Here's the drawing with two shaded views (mm, measured from the low corner). I have some questions. A direction names the side the tool comes from. Round coordinates to 2 decimals unless told otherwise and drop trailing zeros. Loops run counter-clockwise (first coordinate to the right, second up) from the corner with the lowest first, then second, coordinate; pieces in that order, holes last. Notation, with made-up numbers: (43, 0.5) -> (86, 0.5) arc R32 cw to (86, 34.5) -> close; hole circle Ø1 at (78.25, 88.5). An arc over 180 degrees is marked (long way). Write each question's results on one line, items separated by ' | '. Start each with the question number.
1) Imagine slicing it at C-C, the plane y = 3.75. List the corners of the cut face in (x, z) for me.
2) Imagine slicing it at D-D, the plane z = 2.75. List the corners of the cut face in (x, y) for me (1 decimal).
3) Imagine slicing it at B-B, the plane x = 57. List the corners of the cut face in (y, z) for me.
4) We'd pull the mould along Z, two halves only. Please class the marked faces 4, 5, 6 and 7: pulls with the +Z half, pulls with the -Z half, needs draft (parallel to the pull), parting line crosses it, or undercut.
5) Which directions (+Z, -Z, +X, -X, +Y, -Y) give clear straight access to the entire face, cutting with the end or side of a thin tool? Please do the marked faces 1, 2 and 3.
6) Imagine slicing it at A-A, the plane y = 16.5. List the corners of the cut face in (x, z) for me, plus the area to 3 significant figures.
7) If I drill on probe 1 along Z at (x, y) = (19, 6.75); probe 2 along Y at (x, z) = (15, 4); probe 3 along Z at (x, y) = (62.5, 5.5), over which ranges is the centre line in solid material (lowest first)?
8) For P1, Ø2.5, axis at x = 4, z = 6.5, coming from the -Y side; P2, Ø1.6, axis at y = 14, z = 5, coming from the -X side; P3, Ø2, axis at x = 38.5, z = 4.5, coming from the -Y side; P4, Ø2, axis at x = 48, y = 21.5, coming from the +Z side, each with a flat end and sliding along its axis, tell me the tip position at first contact or that it passes through.
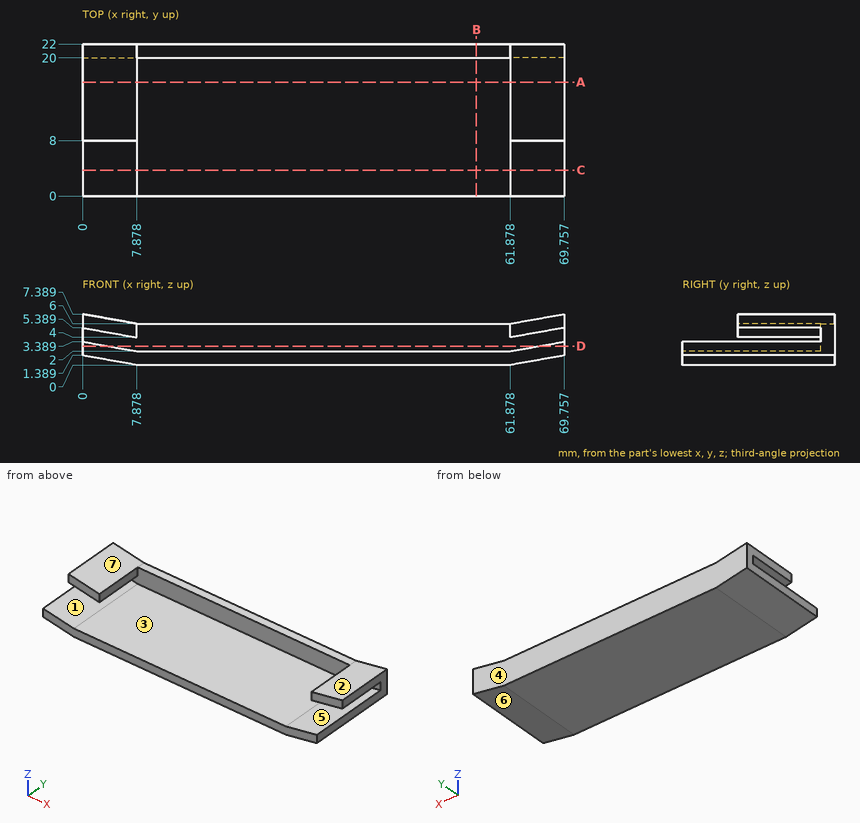
Checked values:
1) outline: (0, 1.39) -> (7.88, 0) -> (61.88, 0) -> (69.76, 1.39) -> (69.76, 3.39) -> (61.88, 2) -> (7.88, 2) -> (0, 3.39) -> close
2) outline: (0, 0) -> (3.6, 0) -> (3.6, 20) -> (66.1, 20) -> (66.1, 0) -> (69.8, 0) -> (69.8, 22) -> (0, 22) -> close
3) outline: (0, 0) -> (22, 0) -> (22, 6) -> (20, 6) -> (20, 2) -> (0, 2) -> close
4) face 4: needs draft | face 5: undercut | face 6: pulls with the -Z half | face 7: pulls with the +Z half
5) face 1: -Y | face 2: +Z, +Y, -Y | face 3: +Z, -Y
6) outline: (0, 1.39) -> (7.88, 0) -> (61.88, 0) -> (69.76, 1.39) -> (69.76, 3.39) -> (61.88, 2) -> (7.88, 2) -> (0, 3.39) -> close; (0, 5.39) -> (7.88, 4) -> (7.88, 6) -> (0, 7.39) -> close; (61.88, 4) -> (69.76, 5.39) -> (69.76, 7.39) -> (61.88, 6) -> close | area: 171 mm^2
7) probe 1: 0 to 2 | probe 2: 20 to 22 | probe 3: 0.11 to 2.11
8) P1: y = 8 | P2: x = 0 | P3: y = 20 | P4: z = 6
